Can you work these out from the model? Positions are in its coordinate system, mm. Round coordinates to 2 decimals unless told otherwise and drop trailing zeros. Order: outer loops, then holes, each group sorted by start corner. A loop starts at its lowest first (then second) coordinate and runs counter-clockwise, first axis right, second up.
Q1. If we section it at B-B (y = 20): Please give me the cut outline in (x, z).
Q2. If we section it at D-D (z = 2.3): Please give me the cut outline in (x, y).
Q3. If I drill on line 1 (Y direction, x = 52, z = 2.3); line 2 (X direction, y = 19.5, z = 3.4); line 3 (X direction, y = 31.5, z = 0.9), over which ranges is the centre line in solid material (lowest first)?
Q4. We'd pull the mould along Y, two halves only. Please class faces 1 (the face through (30, 0, 2)), 2 (the face through (43, 20, 0)), 3 (the face through (53.34, 32.11, 2.54)), 4 (the face through (30, 40, 2)): pulls with the +Y half, pulls with the -Y half, needs draft (parallel to the pull), parting line crosses it, or undercut.
Q5. If we section it at C-C (x = 30): Please give me the cut outline in (y, z).
Q6. If we section it at A-A (x = 8): Please give me the cut outline in (y, z).
from build123d import *

# Parameters (mm, degrees)
SKETCH1_W           = 60
SKETCH1_H           = 40
BOSS_EXTRUDE1_DEPTH = 5
SKETCH2_R           = 12.5
CUT_EXTRUDE1_DEPTH  = 5
SKETCH3_R           = 2.5
CUT_EXTRUDE2_DEPTH  = 10


with BuildPart() as part:
    # Sketch1 → Boss-Extrude1 (new body)
    with BuildSketch(Plane.XY):
        with Locations((30, 20)):
            Rectangle(SKETCH1_W, SKETCH1_H)
    extrude(amount=BOSS_EXTRUDE1_DEPTH)

    # Sketch2 → Cut-Extrude1 (cut)
    with BuildSketch(Plane.XY.offset(5)):
        with Locations((30, 20)):
            Circle(SKETCH2_R)
    extrude(amount=-CUT_EXTRUDE1_DEPTH, mode=Mode.SUBTRACT)

    # Sketch3 → Cut-Extrude2 (cut)
    with BuildSketch(Plane.XY.offset(5)):
        with Locations((8, 30)):
            Circle(SKETCH3_R)
        with Locations((8, 10)):
            Circle(SKETCH3_R)
        with Locations((52, 10)):
            Circle(SKETCH3_R)
        with Locations((52, 30)):
            Circle(SKETCH3_R)
    extrude(amount=-CUT_EXTRUDE2_DEPTH, mode=Mode.SUBTRACT)


solid = part.part
Solution:
1. outline: (0, 0) - (17.5, 0) - (17.5, 5) - (0, 5) - close; (42.5, 0) - (60, 0) - (60, 5) - (42.5, 5) - close
2. outline: (0, 0) - (60, 0) - (60, 40) - (0, 40) - close; hole circle Ø5 at (8, 10); hole circle Ø5 at (8, 30); hole circle Ø25 at (30, 20); hole circle Ø5 at (52, 10); hole circle Ø5 at (52, 30)
3. line 1: y = 0 to 7.5, 12.5 to 27.5, 32.5 to 40
3. line 2: x = 0 to 17.51, 42.49 to 60
3. line 3: x = 0 to 6, 10 to 25.1, 34.9 to 50, 54 to 60
4. face 1: pulls with the -Y half
4. face 2: needs draft
4. face 3: undercut
4. face 4: pulls with the +Y half
5. outline: (0, 0) - (7.5, 0) - (7.5, 5) - (0, 5) - close; (32.5, 0) - (40, 0) - (40, 5) - (32.5, 5) - close
6. outline: (0, 0) - (7.5, 0) - (7.5, 5) - (0, 5) - close; (12.5, 0) - (27.5, 0) - (27.5, 5) - (12.5, 5) - close; (32.5, 0) - (40, 0) - (40, 5) - (32.5, 5) - close
